Could you check a few things on this model? Use its own coordinates, in mm. A direction names the side the tool comes from. Coordinates: 2 decimals unless noted, no trailing zeros. Loops run counter-clockwise (first coordinate to the right, second up) from the corner with the lowest first, then second, coordinate; pieces in that order, holes last. Notation, with made-up numbers: M 62,5.5 L 87,5.5 A18 cw 87,18.5 Z; hole C 54.5,-2.75 d8. An arc over 180 degrees is marked long. Write each question's results on one line, items separated by ' | '.
```python
from build123d import *

# Parameters (mm, degrees)
BASE_FLANGE1_DEPTH = 150
CUT_EXTRUDE2_DEPTH = 163.385344166
SKETCH5_W          = 35
SKETCH5_H          = 2.2366
CUT_EXTRUDE3_DEPTH = 169.696472992
FILLET1_R          = 5


# Sheet-metal steps are written as plain solids
with BuildPart() as part:
    # Sketch1 → Base-Flange1 (new body)
    with BuildSketch(Plane.XY):
        with BuildLine():
            Line((-35.5, -25), (34.7634, -25))
            ThreePointArc((34.7634, -25), (35.284254855, -24.784254855), (35.5, -24.2634))
            Line((35.5, -24.2634), (35.5, 25))
            Line((35.5, 25), (37, 25))
            Line((37, 25), (37, -24.2634))
            ThreePointArc((37, -24.2634), (36.344915027, -25.844915027), (34.7634, -26.5))
            Line((34.7634, -26.5), (-35.5, -26.5))
            Line((-35.5, -26.5), (-35.5, -25))
        make_face()
    extrude(amount=BASE_FLANGE1_DEPTH)

    # Sketch4 → Cut-Extrude2 (cut, through all)
    with BuildSketch(Plane(origin=(0, -25, 0), x_dir=(1, 0, 0), z_dir=(0, 1, 0))):
        with BuildLine():
            Line((-20.5, -102.45), (-5.5, -102.45))
            ThreePointArc((-5.5, -102.45), (-2.95, -105), (-5.5, -107.55))
            Line((-5.5, -107.55), (-20.5, -107.55))
            ThreePointArc((-20.5, -107.55), (-23.05, -105), (-20.5, -102.45))
        make_face()
        with BuildLine():
            Line((-20.5, -42.45), (-5.5, -42.45))
            ThreePointArc((-5.5, -42.45), (-2.95, -45), (-5.5, -47.55))
            Line((-5.5, -47.55), (-20.5, -47.55))
            ThreePointArc((-20.5, -47.55), (-23.05, -45), (-20.5, -42.45))
        make_face()
    extrude(amount=-CUT_EXTRUDE2_DEPTH, mode=Mode.SUBTRACT)

    # Sketch5 → Cut-Extrude3 (cut, through all)
    with BuildSketch(Plane.ZY.offset(35.5)):
        with Locations((132.5, -25.3817)):
            Rectangle(SKETCH5_W, SKETCH5_H)
        with Locations((17.5, -25.3817)):
            Rectangle(SKETCH5_W, SKETCH5_H)
    extrude(amount=-CUT_EXTRUDE3_DEPTH, mode=Mode.SUBTRACT)

    # Fillet1
    fillet1_edges = [part.edges().sort_by_distance(p)[0] for p in [
        (36.25, -24.2634, 0),
        (36.25, -24.2634, 150),
        (36.25, 25, 150),
        (-35.5, -25.75, 115),
        (36.25, 25, 0),
        (-35.5, -25.75, 35),
    ]]
    fillet(fillet1_edges, radius=FILLET1_R)


solid = part.part
```
(1) Imagine slicing it at C-C, the plane z = 67.5. List the corners of the cut face in (x, y) for me, and give its area (3 significant figures).
Reported:
outline: M -35.5,-26.5 L 34.76,-26.5 A2.24 ccw 37,-24.26 L 37,25 L 35.5,25 L 35.5,-24.26 A0.74 cw 34.76,-25 L -35.5,-25 Z | area: 183 mm2
(2) Imagine slicing it at B-B, the plane z = 105. List the corners of the cut face in (x, y) for me, and give its area (3 significant figures).
Reported:
outline: M -35.5,-26.5 L -23.05,-26.5 L -23.05,-25 L -35.5,-25 Z; M -2.95,-26.5 L 34.76,-26.5 A2.24 ccw 37,-24.26 L 37,25 L 35.5,25 L 35.5,-24.26 A0.74 cw 34.76,-25 L -2.95,-25 Z | area: 153 mm2
(3) Please list where these lines run through material, in increasing order: probe 1 along X at (y, z) = (18.5, 61); probe 2 along Y at (x, z) = (0.5, 106.5). Write a range as from..to.
Reported:
probe 1: x = 35.5..37 | probe 2: y = -26.5..-25
(4) Imagine slicing it at A-A, the plane x = -8.5. List the corners of the cut face in (y, z) for me, and give its area (3 significant figures).
Reported:
outline: M -26.5,35 L -25,35 L -25,42.45 L -26.5,42.45 Z; M -26.5,47.55 L -25,47.55 L -25,102.45 L -26.5,102.45 Z; M -26.5,107.55 L -25,107.55 L -25,115 L -26.5,115 Z | area: 105 mm2
(5) Which directions (+Z, -Z, +X, -X, +Y, -Y) give clear straight access to the entire face, cutting with the end or side of a thin tool? Please do faces 1 (the cylindrical face through (-34, -25.74, 36.43)), 2 (the flat face through (35.5, 0, 74)).
Reported:
face 1: -Z, -X, +Y, -Y | face 2: +Z, -Z, -X, +Y
(6) Imagine slicing it at D-D, the plane y = -10.5. List the corners of the cut face in (x, z) for me, and give its area (3 significant figures).
Reported:
outline: M 35.5,0 L 37,0 L 37,150 L 35.5,150 Z | area: 225 mm2
(7) Will these pins go through, and if not, where does the flat tip stop? P1, Ø24.5, axis at y = -1, z = 112, coming from the -X side; P2, Ø1.8, axis at x = -2, y = -25.5, coming from the +Z side; P3, Ø1.6, axis at x = -16, y = -25.5, coming from the -Z side.
Reported:
P1: stops at x = 35.5 | P2: stops at z = 115 | P3: stops at z = 35
